from build123d import *

# Parameters (mm, degrees)
SKETCH1_W            = 40
SKETCH1_H            = 20
SKETCH1_W_2          = 35
SKETCH1_H_2          = 15
BOSS_EXTRUDE1_DEPTH  = 1600
SKETCH2_W            = 40
SKETCH2_H            = 20
SKETCH2_W_2          = 35
SKETCH2_H_2          = 15
BOSS_EXTRUDE3_DEPTH  = 1000
SKETCH3_W            = 40
SKETCH3_H            = 20
SKETCH3_W_2          = 35
SKETCH3_H_2          = 15
BOSS_EXTRUDE4_DEPTH  = 1600
SKETCH4_W            = 20
SKETCH4_H            = 40
SKETCH4_W_2          = 15
SKETCH4_H_2          = 35
BOSS_EXTRUDE5_DEPTH  = 700
SKETCH5_W            = 40
SKETCH5_H            = 20
SKETCH5_W_2          = 35
SKETCH5_H_2          = 15
BOSS_EXTRUDE6_DEPTH  = 1600
SKETCH7_W            = 40
SKETCH7_H            = 20
SKETCH7_W_2          = 35
SKETCH7_H_2          = 15
BOSS_EXTRUDE7_DEPTH  = 200
SKETCH10_W           = 40
SKETCH10_H           = 20
SKETCH10_W_2         = 35
SKETCH10_H_2         = 15
BOSS_EXTRUDE9_DEPTH  = 200
SKETCH11_W           = 40
SKETCH11_H           = 20
SKETCH11_W_2         = 35
SKETCH11_H_2         = 15
BOSS_EXTRUDE10_DEPTH = 1600
SKETCH12_W           = 20
SKETCH12_H           = 40
SKETCH12_W_2         = 15
SKETCH12_H_2         = 35
BOSS_EXTRUDE11_DEPTH = 700
SKETCH14_R           = 5
BOSS_EXTRUDE13_DEPTH = 1550


with BuildPart() as part:
    # Sketch1 → Boss-Extrude1 (new body)
    with BuildSketch(Plane.XY):
        Rectangle(SKETCH1_W, SKETCH1_H)
        Rectangle(SKETCH1_W_2, SKETCH1_H_2, mode=Mode.SUBTRACT)
    extrude(amount=BOSS_EXTRUDE1_DEPTH)

    # Sketch2 → Boss-Extrude3 (add)
    # profile 1 of 2: a face of its own
    with BuildSketch(Plane(origin=(20, 0, 0), x_dir=(0, 0, -1), z_dir=(1, 0, 0))):
        with Locations((-1580, 0)):
            Rectangle(SKETCH2_W, SKETCH2_H)
        with Locations((-1580, 0)):
            Rectangle(SKETCH2_W_2, SKETCH2_H_2, mode=Mode.SUBTRACT)
    # profile 2 of 2: a face of its own
    with BuildSketch(Plane(origin=(20, 0, 0), x_dir=(0, 0, -1), z_dir=(1, 0, 0))):
        with Locations((-20, 0)):
            Rectangle(SKETCH2_W, SKETCH2_H)
        with Locations((-20, 0)):
            Rectangle(SKETCH2_W_2, SKETCH2_H_2, mode=Mode.SUBTRACT)
    extrude(amount=BOSS_EXTRUDE3_DEPTH)

    # Sketch3 → Boss-Extrude4 (add)
    with BuildSketch(Plane.XY.offset(1600)):
        with Locations((1040, 0)):
            Rectangle(SKETCH3_W, SKETCH3_H)
        with Locations((1040, 0)):
            Rectangle(SKETCH3_W_2, SKETCH3_H_2, mode=Mode.SUBTRACT)
    extrude(amount=-BOSS_EXTRUDE4_DEPTH)

    # Sketch4 → Boss-Extrude5 (add)
    # profile 1 of 4: a face of its own
    with BuildSketch(Plane.XZ.offset(10)):
        with Locations((1050, 1580)):
            Rectangle(SKETCH4_W, SKETCH4_H)
        with Locations((1050, 1580)):
            Rectangle(SKETCH4_W_2, SKETCH4_H_2, mode=Mode.SUBTRACT)
    # profile 2 of 4: a face of its own
    with BuildSketch(Plane.XZ.offset(10)):
        with Locations((1050, 20)):
            Rectangle(SKETCH4_W, SKETCH4_H)
        with Locations((1050, 20)):
            Rectangle(SKETCH4_W_2, SKETCH4_H_2, mode=Mode.SUBTRACT)
    # profile 3 of 4: a face of its own
    with BuildSketch(Plane.XZ.offset(10)):
        with Locations((-10, 20)):
            Rectangle(SKETCH4_W, SKETCH4_H)
        with Locations((-10, 20)):
            Rectangle(SKETCH4_W_2, SKETCH4_H_2, mode=Mode.SUBTRACT)
    # profile 4 of 4: a face of its own
    with BuildSketch(Plane.XZ.offset(10)):
        with Locations((-10, 1580)):
            Rectangle(SKETCH4_W, SKETCH4_H)
        with Locations((-10, 1580)):
            Rectangle(SKETCH4_W_2, SKETCH4_H_2, mode=Mode.SUBTRACT)
    extrude(amount=BOSS_EXTRUDE5_DEPTH)

    # Sketch5 → Boss-Extrude6 (add)
    # profile 1 of 3: a face of its own
    with BuildSketch(Plane.XY.offset(1600)):
        with Locations((250, -20)):
            Rectangle(SKETCH5_W, SKETCH5_H)
        with Locations((250, -20)):
            Rectangle(SKETCH5_W_2, SKETCH5_H_2, mode=Mode.SUBTRACT)
    # profile 2 of 3: a face of its own
    with BuildSketch(Plane.XY.offset(1600)):
        with Locations((500, -20)):
            Rectangle(SKETCH5_W, SKETCH5_H)
        with Locations((500, -20)):
            Rectangle(SKETCH5_W_2, SKETCH5_H_2, mode=Mode.SUBTRACT)
    # profile 3 of 3: a face of its own
    with BuildSketch(Plane.XY.offset(1600)):
        with Locations((750, -20)):
            Rectangle(SKETCH5_W, SKETCH5_H)
        with Locations((750, -20)):
            Rectangle(SKETCH5_W_2, SKETCH5_H_2, mode=Mode.SUBTRACT)
    extrude(amount=-BOSS_EXTRUDE6_DEPTH)

    # Sketch7 → Boss-Extrude7 (add)
    # profile 1 of 2: a face of its own
    with BuildSketch(Plane(origin=(1060, 0, 0), x_dir=(0, 0, -1), z_dir=(1, 0, 0))):
        with Locations((-1580, 0)):
            Rectangle(SKETCH7_W, SKETCH7_H)
        with Locations((-1580, 0)):
            Rectangle(SKETCH7_W_2, SKETCH7_H_2, mode=Mode.SUBTRACT)
    # profile 2 of 2: a face of its own
    with BuildSketch(Plane(origin=(1060, 0, 0), x_dir=(0, 0, -1), z_dir=(1, 0, 0))):
        with Locations((-20, 0)):
            Rectangle(SKETCH7_W, SKETCH7_H)
        with Locations((-20, 0)):
            Rectangle(SKETCH7_W_2, SKETCH7_H_2, mode=Mode.SUBTRACT)
    extrude(amount=BOSS_EXTRUDE7_DEPTH)

    # Sketch10 → Boss-Extrude9 (add)
    # profile 1 of 2: a face of its own
    with BuildSketch(Plane.ZY.offset(20)):
        with Locations((20, 0)):
            Rectangle(SKETCH10_W, SKETCH10_H)
        with Locations((20, 0)):
            Rectangle(SKETCH10_W_2, SKETCH10_H_2, mode=Mode.SUBTRACT)
    # profile 2 of 2: a face of its own
    with BuildSketch(Plane.ZY.offset(20)):
        with Locations((1580, 0)):
            Rectangle(SKETCH10_W, SKETCH10_H)
        with Locations((1580, 0)):
            Rectangle(SKETCH10_W_2, SKETCH10_H_2, mode=Mode.SUBTRACT)
    extrude(amount=BOSS_EXTRUDE9_DEPTH)

    # Sketch11 → Boss-Extrude10 (add)
    # profile 1 of 2: a face of its own
    with BuildSketch(Plane(origin=(0, 0, 0), x_dir=(-1, 0, 0), z_dir=(0, 0, -1))):
        with Locations((240, 0)):
            Rectangle(SKETCH11_W, SKETCH11_H)
        with Locations((240, 0)):
            Rectangle(SKETCH11_W_2, SKETCH11_H_2, mode=Mode.SUBTRACT)
    # profile 2 of 2: a face of its own
    with BuildSketch(Plane(origin=(0, 0, 0), x_dir=(-1, 0, 0), z_dir=(0, 0, -1))):
        with Locations((-1280, 0)):
            Rectangle(SKETCH11_W, SKETCH11_H)
        with Locations((-1280, 0)):
            Rectangle(SKETCH11_W_2, SKETCH11_H_2, mode=Mode.SUBTRACT)
    extrude(amount=-BOSS_EXTRUDE10_DEPTH)

    # Sketch12 → Boss-Extrude11 (add)
    # profile 1 of 4: a face of its own
    with BuildSketch(Plane.XZ.offset(10)):
        with Locations((1290, 20)):
            Rectangle(SKETCH12_W, SKETCH12_H)
        with Locations((1290, 20)):
            Rectangle(SKETCH12_W_2, SKETCH12_H_2, mode=Mode.SUBTRACT)
    # profile 2 of 4: a face of its own
    with BuildSketch(Plane.XZ.offset(10)):
        with Locations((-250, 20)):
            Rectangle(SKETCH12_W, SKETCH12_H)
        with Locations((-250, 20)):
            Rectangle(SKETCH12_W_2, SKETCH12_H_2, mode=Mode.SUBTRACT)
    # profile 3 of 4: a face of its own
    with BuildSketch(Plane.XZ.offset(10)):
        with Locations((1290, 1580)):
            Rectangle(SKETCH12_W, SKETCH12_H)
        with Locations((1290, 1580)):
            Rectangle(SKETCH12_W_2, SKETCH12_H_2, mode=Mode.SUBTRACT)
    # profile 4 of 4: a face of its own
    with BuildSketch(Plane.XZ.offset(10)):
        with Locations((-250, 1580)):
            Rectangle(SKETCH12_W, SKETCH12_H)
        with Locations((-250, 1580)):
            Rectangle(SKETCH12_W_2, SKETCH12_H_2, mode=Mode.SUBTRACT)
    extrude(amount=BOSS_EXTRUDE11_DEPTH)

    # Sketch14 → Boss-Extrude13 (add)
    with BuildSketch(Plane(origin=(0, 0, 1560), x_dir=(-1, 0, 0), z_dir=(0, 0, -1))):
        with Locations(Location((-1230, 0, 0), (0, 0, 180))):
            Circle(SKETCH14_R)
        with Locations(Location((-1090, 0, 0), (0, 0, 180))):
            Circle(SKETCH14_R)
        with Locations((50, 0)):
            Circle(SKETCH14_R)
        with Locations((190, 0)):
            Circle(SKETCH14_R)
    extrude(amount=BOSS_EXTRUDE13_DEPTH)


solid = part.part
Geometry: final body of the model. Coordinates: model frame, mm. A direction names the side the tool comes from. Round coordinates to 2 decimals unless told otherwise and drop trailing zeros. Order: outer loops, then holes, each group sorted by start corner. A loop starts at its lowest first (then second) coordinate and runs counter-clockwise, first axis right, second up.
Q1. Access query for faces 1 (the face through (227, -2, 0)), 2 (the face through (750, -10, 811)), 3 (the face through (1040, -355, 1580)). Directions: +Z, -Z, +X, -X, +Y, -Y. A direction counts if a zero-diameter tool reaches every point of the face in a straight line with its end or side. Return the directions, or none.
Result sheet:
face 1: -Z, +X, -X, +Y, -Y
face 2: +Y
face 3: +Z, -Z, -Y
Q2. Section B-B, the plane z = 540. Give the number of separate pieces and of enclosed holes in the cut face, and give its area (3 significant figures).
Result sheet:
separate pieces: 11
enclosed holes: 7
area: 2,240 mm2
Q3. Mould query, pull axis X, two halves, no side actions, for faces 4 (the face through (1300, -2, 796)), 5 (the face through (624, -10, 1580)), 6 (the face through (250, -10, 811)), 7 (the face through (1044, 10, 796)). Classes: released by +X, released by -X, zero draft, split by the parting line, or undercut.
Result sheet:
face 4: released by +X
face 5: undercut
face 6: undercut
face 7: zero draft
Q4. Material intervals for probe 1 along X at (y, z) = (-29, 465.5); probe 2 along Y at (x, z) = (15, 69.5), sorted ascending.
Result sheet:
probe 1: x = 230 to 270, 480 to 520, 730 to 770
probe 2: y = -10 to -7.5, 7.5 to 10
Q5. Pin query (flat end, axial travel): pin 1 (7.5 mm diameter, centred on x = -7.5, z = 16.5, fed in from -Y); pin 2 (11 mm diameter, centred on x = 1229, y = -1, fed in from -Z); pin 3 (6 mm diameter, centred on x = 508.5, z = 417, fed in from -Y). Return the tip coordinate at first contact, or that it passes through.
Result sheet:
pin 1: stops at y = -10
pin 2: stops at z = 0
pin 3: stops at y = -30
Q6. Section A-A, the plane x = 320. Output: boundary loops of the cut face in (y, z).
Result sheet:
outline: (-10, 0) - (10, 0) - (10, 40) - (-10, 40) - close; (-10, 1560) - (10, 1560) - (10, 1600) - (-10, 1600) - close; hole (-7.5, 2.5) - (7.5, 2.5) - (7.5, 37.5) - (-7.5, 37.5) - close; hole (-7.5, 1562.5) - (7.5, 1562.5) - (7.5, 1597.5) - (-7.5, 1597.5) - close
